```python
from build123d import *

# Parameters (mm, degrees)
F0_R     = 2.5
F1_DEPTH = 3


with BuildPart() as f1:
    # F0 (on Front) → F1 (new body)
    with BuildSketch(Plane.XZ):
        with BuildLine():
            Line((-40, -6), (0, -6))
            ThreePointArc((0, -6), (6, 0), (0, 6))
            Line((0, 6), (-44.367643, 6))
            Line((-44.367643, 6), (-59.688532, -6.855752))
            ThreePointArc((-59.688532, -6.855752), (-88.934737, -66.948807), (-63.741269, -128.850383))
            Line((-63.741269, -128.850383), (-58.484232, -123.280056))
            ThreePointArc((-58.484232, -123.280056), (-80.29366, -70.359314), (-55.320889, -18.855752))
            Line((-55.320889, -18.855752), (-40, -6))
        make_face()
        with Locations((-40, 0)):
            Circle(F0_R, mode=Mode.SUBTRACT)
        Circle(F0_R, mode=Mode.SUBTRACT)
    extrude(amount=F1_DEPTH)


solid = f1.part
```
The listing builds one solid part. Answer for the finished solid, in the listing's coordinates (mm). A direction names the side the tool comes from. Round coordinates to 2 decimals unless told otherwise and drop trailing zeros. Write each loop counter-clockwise with the first axis right and the second up, starting at its lowest first coordinate (ties: lowest second). Pieces come first, ordered by that corner, then holes. Notation, with made-up numbers: (29.25, 50.25) -> (53.25, 50.25) arc R28 ccw to (53.25, 69.25) -> close; hole circle Ø8 at (-2, 18.25). An arc over 180 degrees is marked (long way). Write item = value, one per line.
1) Section B-B on z = 0 is taken. Write down the section's boundary in (x, y).
Check values:
outline = (-51.52, -3) -> (-42.5, -3) -> (-42.5, 0) -> (-51.52, 0) -> close; (-37.5, -3) -> (-2.5, -3) -> (-2.5, 0) -> (-37.5, 0) -> close; (2.5, -3) -> (6, -3) -> (6, 0) -> (2.5, 0) -> close
2) Section D-D on z = -80 is taken. Write down the section's boundary in (x, y).
Check values:
outline = (-88.33, -3) -> (-79.92, -3) -> (-79.92, 0) -> (-88.33, 0) -> close
3) Straight lines are drawn through the part: line 1 along Z through (x, y) = (-40, -1.2); line 2 along X through (y, z) = (-0.6, -2); line 3 along Z through (x, y) = (-9, -1.95). For each, find the intervals that lie inside material, in ascending order. Write a range as [from, to].
Check values:
line_1 = [-6, -2.5], [2.5, 6]
line_2 = [-53.9, -41.5], [-38.5, -1.5], [1.5, 5.66]
line_3 = [-6, 6]
4) Section C-C on x = -18 is taken. Write down the section's boundary in (y, z).
Check values:
outline = (-3, -6) -> (0, -6) -> (0, 6) -> (-3, 6) -> close
5) For a pull along Z with two mould halves and no side action, classify faces 3 (the cylindrical face through (-88.897, -1.479, -65.986)), 4 (the flat face through (-22, -1, 6)), 5 (the cylindrical face through (-0.54, -1.48, -2.44)) as released by +Z, released by -Z, zero draft, split by the parting line, or undercut.
Check values:
face_3 = split by the parting line
face_4 = released by +Z
face_5 = undercut
6) Which of the six approach directions +Z, -Z, +X, -X, +Y, -Y give full straight-line access (tool end or side, diameter ignored) to faces 1 (the flat face through (-51.921, -1.479, -0.338)), 2 (the flat face through (-20, -1, -6))?
Check values:
face_1 = +Z, -X, +Y, -Y
face_2 = -Z, +X, +Y, -Y
7) Given pin 1 (1.5 mm diameter, centred on y = -0.5, z = -78, fed in from +X); pin 2 (1.5 mm diameter, centred on y = -0.5, z = -53.5, fed in from -X); pin 3 (8 mm diameter, centred on x = -40, z = 0, fed in from -Y), each flat-ended and moving along its own axis, determine where each tip first touches the part or whether it passes through.
Check values:
pin_1 = -80.04
pin_2 = -87.52
pin_3 = -3
8) Section A-A on y = -2.5 is taken. Write down the section's boundary in (x, z), plus the area to 3 significant figures.
Check values:
outline = (-63.74, -128.85) -> (-58.48, -123.28) arc R70 cw to (-55.32, -18.86) -> (-40, -6) -> (0, -6) arc R6 ccw to (0, 6) -> (-44.37, 6) -> (-59.69, -6.86) arc R82 ccw to start; hole circle Ø5 at (-40, 0); hole circle Ø5 at (0, 0)
area = 1,930 mm²
